Source: CAD feature listing. Evaluate the final solid. Frame: model axes, mm. A direction names the side the tool comes from. Give positions to 0.01 mm unless a question says otherwise; leave off trailing zeros. Order: outer loops, then holes, each group sorted by start corner. A loop starts at its lowest first (then second) coordinate and runs counter-clockwise, first axis right, second up. Notation, with made-up numbers: (82, 54) - (138, 54) arc R26 cw to (138, 72) - close; hole circle Ø7 at (46.25, -24). An arc over 180 degrees is marked (long way). Answer as CSV lines item,"result".
Autodesk Inventor part; units mm, degrees
ref_plane "YZ Plane" through (0, 0, 0) normal (1, 0, 0) x (0, 1, 0)
ref_plane "XZ Plane" through (0, 0, 0) normal (0, 1, 0) x (-1, 0, 0)
ref_plane "XY Plane" through (0, 0, 0) normal (0, 0, 1) x (1, 0, 0)
sketch "Sketch1" plane through (0, 0, 0) normal (0, 0, 1) x (1, 0, 0)
  line L0 (0, 0) -> (330, 0)
  line L1 (330, 0) -> (330, 510)
  line L2 (330, 510) -> (0, 510)
  line L3 (0, 510) -> (0, 0)
  dimension "d0" = 330
  dimension "d1" = 510
extrude "Extrusion1" add sketch "Sketch1" along normal blind 150
sketch "Sketch2" plane through (0, 0, 0) normal (0, -1, 0) x (1, 0, 0)
  circle A0 centre (165, -304.672) radius 315
  line L0 (85, 0) -> (245, 0)
  line L1 (0, 0) -> (330, 0)
  circle A1 centre (165, -304.672) radius 317
  point P0 (165, 0)
  point P1 (165, 0)
  dimension "d4" = 630
  dimension "d8" = 160
  dimension "d9" = 2
extrude "Extrusion2" cut sketch "Sketch2" against normal through all
sketch "Sketch3" plane through (0, 0, 150) normal (0, 0, 1) x (1, 0, 0)
  line L0 (0, 0) -> (330, 0)
  line L1 (330, 0) -> (330, 510)
  line L2 (330, 510) -> (0, 510)
  line L3 (0, 510) -> (0, 0)
  line L4 (10, 10) -> (320, 10)
  line L5 (320, 10) -> (320, 500)
  line L6 (320, 500) -> (10, 500)
  line L7 (10, 500) -> (10, 10)
  dimension "d10" = 10
extrude "Extrusion3" cut sketch "Sketch3" against normal blind 130 contours L7 L6 L5 L4
sketch "Sketch4" plane through (0, 0, 20) normal (0, 0, 1) x (1, 0, 0)
  line L0 (10, 500) -> (320, 500) construction
  line L1 (85, 500) -> (245, 500) construction
  line L2 (245, 500) -> (245, 10) construction
  line L3 (245, 10) -> (85, 10) construction
  line L4 (85, 10) -> (85, 500) construction
  line L5 (320, 10) -> (10, 10) construction
  line L6 (85, 500) -> (245, 500) construction
  line L7 (245, 500) -> (245, 455) construction
  line L8 (245, 455) -> (85, 455) construction
  line L9 (85, 455) -> (85, 500) construction
  line L10 (85, 455) -> (245, 455) construction
  line L11 (245, 455) -> (245, 400) construction
  line L12 (245, 400) -> (85, 400) construction
  line L13 (85, 400) -> (85, 455) construction
  line L14 (85, 400) -> (245, 400) construction
  line L15 (245, 400) -> (245, 345) construction
  line L16 (245, 345) -> (85, 345) construction
  line L17 (85, 345) -> (85, 400) construction
  line L18 (85, 345) -> (245, 345) construction
  line L19 (245, 345) -> (245, 290) construction
  line L20 (245, 290) -> (85, 290) construction
  line L21 (85, 290) -> (85, 345) construction
  line L22 (85, 290) -> (245, 290) construction
  line L23 (245, 290) -> (245, 235) construction
  line L24 (245, 235) -> (85, 235) construction
  line L25 (85, 235) -> (85, 290) construction
  circle A0 centre (130.3559, 262.5) radius 15
  circle A1 centre (199.6441, 262.5) radius 15
  line L26 (130.3559, 262.5) -> (199.6441, 262.5) construction
  point P0 (0, 0)
  point P1 (165, 500)
  point P2 (165, 500)
  point P3 (165, 262.5)
  point P4 (165, 235)
  point P5 (245, 262.5)
  dimension "d13" = 160
  dimension "d14" = 45
  dimension "d15" = 55
  dimension "d16" = 55
  dimension "d17" = 55
  dimension "d18" = 55
  dimension "d19" = 30
  dimension "d20" = 30
  dimension "d21" = 69.2883
extrude "Extrusion4" cut sketch "Sketch4" against normal through all
properties part number "CA002" material "ABS Plastic"
(1) Cut plane B-B (y = 255). Return loops of the section in (x, z).
Completed:
outline,"(0, 0) - (77.46, 0) arc R317 cw to (117.37, 8.73) - (117.37, 20) - (10, 20) - (10, 150) - (0, 150) - close; (143.35, 11.59) arc R317 cw to (186.65, 11.59) - (186.65, 20) - (143.35, 20) - close; (212.63, 8.73) arc R317 cw to (252.54, 0) - (330, 0) - (330, 150) - (320, 150) - (320, 20) - (212.63, 20) - close"
(2) Cut plane A-A (x = 35.5). Return loops of the section in (y, z), then the cut area to 3 significant figures.
Completed:
outline,"(0, 0) - (510, 0) - (510, 150) - (500, 150) - (500, 20) - (10, 20) - (10, 150) - (0, 150) - close"
area,"12,800 mm²"
(3) Access query for faces 5 (the flat face through (163, 258, 20)), 6 (the cylindrical face through (115.37, 263.16, 15.58)). Directions: +Z, -Z, +X, -X, +Y, -Y. A direction counts if a zero-diameter tool reaches every point of the face in a straight line with its end or side. Return the directions, or none.
Completed:
face 5,"+Z"
face 6,"+Z, -Z"
(4) Cut plane C-C (z = 128). Return loops of the section in (x, y), then the cut area to 3 significant figures.
Completed:
outline,"(0, 0) - (330, 0) - (330, 510) - (0, 510) - close; hole (10, 10) - (320, 10) - (320, 500) - (10, 500) - close"
area,"16,400 mm²"
(5) Cut plane D-D (x = 134). Return loops of the section in (y, z).
Completed:
outline,"(0, 10.81) - (247.95, 10.81) - (247.95, 20) - (10, 20) - (10, 150) - (0, 150) - close; (277.05, 10.81) - (510, 10.81) - (510, 150) - (500, 150) - (500, 20) - (277.05, 20) - close"
(6) Mould query, pull axis Y, two halves, no side actions, for faces 1 (the flat face through (5, 332, 150)), 2 (the flat face through (10, 258, 86)), 3 (the flat face through (167, 510, 74)), 4 (the cylindrical face through (213.5, 256.75, 15.58)). Classes: released by +Y, released by -Y, zero draft, split by the parting line, or undercut.
Completed:
face 1,"zero draft"
face 2,"undercut"
face 3,"released by +Y"
face 4,"undercut"
(7) Contact query for flat-ended pins moving along their axis: pin 1 (6 mm diameter, centred on x = 200.5, y = 328, fed in from -Z); pin 2 (5 mm diameter, centred on y = 97.5, z = 52, fed in from -X); pin 3 (6 mm diameter, centred on x = 213, y = 449.5, fed in from -Z); pin 4 (8 mm diameter, centred on x = 224.5, y = 363, fed in from -Z). Output: stop coordinate, or through.
Completed:
pin 1,"z = 9.98"
pin 2,"x = 0"
pin 3,"z = 8.2"
pin 4,"z = 5.9"
(8) Ray query, line 1 (X direction, y = 262, z = 13); line 2 (X direction, y = 262, z = 11); line 3 (Y direction, x = 126.5, z = 33.5). Return the intervals inside material, ascending. Write a range as from..to.
Completed:
line 1,"0..115.36, 145.35..184.65, 214.64..330"
line 2,"0..115.36, 214.64..330"
line 3,"0..10, 500..510"
